The listing builds one solid part. Answer for the finished solid, in the listing's coordinates (mm). Coordinates: 2 decimals unless noted, no trailing zeros. Order: outer loops, then holes, each group sorted by start corner. A loop starts at its lowest first (then second) coordinate and runs counter-clockwise, first axis right, second up. Notation, with made-up numbers: M -6.75,79 L 2.25,79 A27 cw 2.25,117 Z; hole C 22,18.5 d10. An arc over 180 degrees is marked long. One line per item, written item: value. Start each with the question number.
Q1. Straight lines are drawn through the part: line 1 along X through (y, z) = (-0.1, 21.5); line 2 along Z through (x, y) = (-1.75, 2.35). For each, find the intervals that lie inside material, in ascending order. Write a range as [from, to].
Q2. Each of these flat-tipped pins is pushed along its axis until it touches: pin 1 Ø2 at (x, z) = (0.5, 11.5) entering from -Y; pin 2 Ø1.5 at (y, z) = (-0.5, 8.5) entering from +X; pin 3 Ø1 at (x, z) = (1.5, 6) entering from -Y; pin 4 Ø2.5 at (x, y) = (0, 0) entering from -Z. Where does it stop, or does it pass through?
Q3. The part is cut by section A-A on x = 0. Give the vertices of the cut face in (y, z) (3 decimals).
Q4. The part is cut by section B-B on y = -1.85. Give the vertices of the cut face in (x, z).
Q5. Determine the mould class of faces 1 (the flat face through (1.4, 0.7, 37)), 2 (the flat face through (1.4, 0.7, 0)), 3 (the cylindrical face through (2.184, 0.688, 18.696)), 4 (the flat face through (0, -2.775, 2)) for opening direction Z: pulls with the +Z half, pulls with the -Z half, needs draft (parallel to the pull), parting line crosses it, or undercut.
Q6. The part is cut by section C-C on z = 21.5. Give the vertices of the cut face in (x, y).
```python
from build123d import *

# Parameters (mm, degrees)
Y_KSEKLIK_EKSTR_ZYON1_DEPTH = 37
KES_EKSTR_ZYON1_START       = -4.5
IZIM2_R                     = 3.29
IZIM2_R_2                   = 2.29
KES_EKSTR_ZYON1_DEPTH       = 28
IZIM3_R                     = 1.35
KES_EKSTR_ZYON2_DEPTH       = 38.242020958


with BuildPart() as part:
    # Çizim1 → Yükseklik-Ekstrüzyon1 (new body)
    with BuildSketch(Plane.XY):
        Polygon((1.602146997, -2.775), (3.204293994, 0), (1.602146997, 2.775), (-1.602146997, 2.775), (-3.204293994, 0), (-1.602146997, -2.775), align=None)
    extrude(amount=Y_KSEKLIK_EKSTR_ZYON1_DEPTH)

    # Çizim2 → Kes-Ekstrüzyon1 (cut)
    with BuildSketch(Plane.XY.offset(37).offset(KES_EKSTR_ZYON1_START)):
        Circle(IZIM2_R)
        Circle(IZIM2_R_2, mode=Mode.SUBTRACT)
    extrude(amount=-KES_EKSTR_ZYON1_DEPTH, mode=Mode.SUBTRACT)

    # Çizim3 → Kes-Ekstrüzyon2 (cut, through all)
    with BuildSketch(Plane(origin=(0, 0, 0), x_dir=(-1, 0, 0), z_dir=(0, 0, -1))):
        Circle(IZIM3_R)
    extrude(amount=-KES_EKSTR_ZYON2_DEPTH, mode=Mode.SUBTRACT)


solid = part.part
```
Output:
1. line 1: x = [-2.29, -1.35], [1.35, 2.29]
1. line 2: z = [0, 4.5], [32.5, 37]
2. pin 1: stops at y = -2.29
2. pin 2: stops at x = 2.29
2. pin 3: stops at y = -2.06
2. pin 4: passes through
3. outline: M -2.775,0 L -1.35,0 L -1.35,37 L -2.775,37 L -2.775,32.5 L -2.29,32.5 L -2.29,4.5 L -2.775,4.5 Z; M 1.35,0 L 2.775,0 L 2.775,4.5 L 2.29,4.5 L 2.29,32.5 L 2.775,32.5 L 2.775,37 L 1.35,37 Z
4. outline: M -2.14,0 L 2.14,0 L 2.14,4.5 L 1.35,4.5 L 1.35,32.5 L 2.14,32.5 L 2.14,37 L -2.14,37 L -2.14,32.5 L -1.35,32.5 L -1.35,4.5 L -2.14,4.5 Z
5. face 1: pulls with the +Z half
5. face 2: pulls with the -Z half
5. face 3: undercut
5. face 4: needs draft
6. outline: C 0,0 d4.58; hole C 0,0 d2.7
